from build123d import *

# Parameters (mm, degrees)
F1_DEPTH = 18
F2_R     = 2
F3_R     = 4


with BuildPart() as f1:
    # F0 (on Front) → F1 (new body)
    with BuildSketch(Plane.XZ):
        Polygon((16.5, 8.5), (16.5, -8.5), (-16.5, -8.5), (-16.5, -10.5), (18.5, -10.5), (18.5, 10.5), (-21.5, 10.5), (-21.5, 8.5), (-20, 8.5), (-18.25, 6), (-16.5, 8.5), align=None)
    extrude(amount=F1_DEPTH)

    # F2
    f2_edges = [f1.edges().sort_by_distance(p)[0] for p in [
        (16.5, -9, 8.5),
        (16.5, -9, -8.5),
    ]]
    fillet(f2_edges, radius=F2_R)

    # F3
    f3_edges = [f1.edges().sort_by_distance(p)[0] for p in [
        (18.5, -9, 10.5),
        (18.5, -9, -10.5),
    ]]
    fillet(f3_edges, radius=F3_R)


solid = f1.part
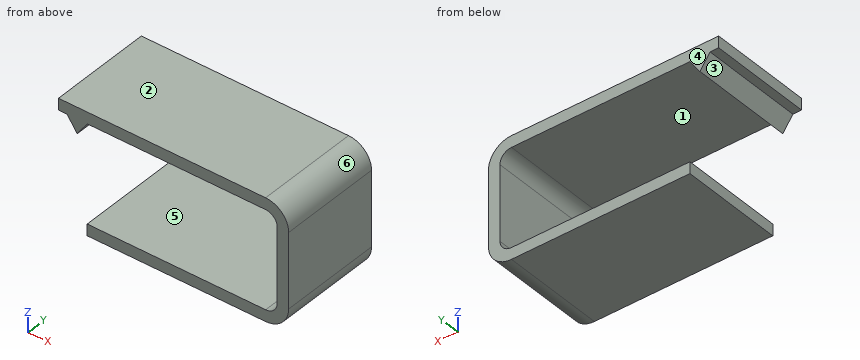
Geometry: final body of the model. Coordinates: model frame, mm. Face numbers are marked on the shaded views. A direction names the side the tool comes from. Round coordinates to 2 decimals unless told otherwise and drop trailing zeros. Write each loop counter-clockwise with the first axis right and the second up, starting at its lowest first coordinate (ties: lowest second). Pieces come first, ordered by that corner, then holes. Notation, with made-up numbers: M 59,-38.5 L 99,-38.5 A20 ccw 99,-31.5 Z; hole C 24,42 d1. An arc over 180 degrees is marked long. Write item = value, one per line.
Item 1: Material intervals for line 1 along Z through (x, y) = (8, -10.25); line 2 along X through (y, z) = (-12.5, -4.75); line 3 along Z through (x, y) = (15.5, -14.75), sorted ascending. Write a range as [from, to].
Findings:
line_1 = [-10.5, -8.5], [8.5, 10.5]
line_2 = [16.5, 18.5]
line_3 = [-10.37, -8.23], [8.23, 10.37]
Item 2: Access query for the marked faces 1 and 2. Directions: +Z, -Z, +X, -X, +Y, -Y. A direction counts if a zero-diameter tool reaches every point of the face in a straight line with its end or side. Return the directions, or none.
Findings:
face_1 = +Y, -Y
face_2 = +Z, +X, -X, +Y, -Y
Item 3: Section query B-B on y = -1.5. Return loops of the section in (x, z).
Findings:
outline = M -21.5,8.5 L -20,8.5 L -18.25,6 L -16.5,8.5 L 14.5,8.5 A2 cw 16.5,6.5 L 16.5,-6.5 A2 cw 14.5,-8.5 L -16.5,-8.5 L -16.5,-10.5 L 14.5,-10.5 A4 ccw 18.5,-6.5 L 18.5,6.5 A4 ccw 14.5,10.5 L -21.5,10.5 Z
Item 4: Pin query (flat end, axial travel): P1, Ø6, axis at y = -3, z = 3.5, coming from the -X side; P2, Ø10.5, axis at y = -11, z = 2.5, coming from the -X side (3 decimals); P3, Ø0.6, axis at y = -12, z = -9.5, coming from the -X side. Return the tip coordinate at first contact, or that it passes through.
Findings:
P1 = -18.6
P2 = -19.475
P3 = -16.5
Item 5: Section query A-A on x = 3.5. Return loops of the section in (y, z), then the cut area to 3 significant figures.
Findings:
outline = M -18,-10.5 L 0,-10.5 L 0,-8.5 L -18,-8.5 Z; M -18,8.5 L 0,8.5 L 0,10.5 L -18,10.5 Z
area = 72.0 mm^2
Item 6: Section query C-C on z = -3. Return loops of the section in (x, y), then the cut area to 3 significant figures.
Findings:
outline = M 16.5,-18 L 18.5,-18 L 18.5,0 L 16.5,0 Z
area = 36.0 mm^2
Item 7: Section query D-D on x = -17. Return loops of the section in (y, z), then the cut area to 3 significant figures.
Findings:
outline = M -18,7.79 L 0,7.79 L 0,10.5 L -18,10.5 Z
area = 48.9 mm^2
Item 8: Pull-direction query (Z, two-part tool) for the marked faces 3, 4, 5 and 6; classes: pulls with the +Z half, pulls with the -Z half, needs draft (parallel to the pull), parting line crosses it, or undercut.
Findings:
face_3 = pulls with the -Z half
face_4 = needs draft
face_5 = undercut
face_6 = pulls with the +Z half
